For this review, take the finished solid that the model builds, in its own axes (mm). Coordinates: 2 decimals unless noted, no trailing zeros. Loops run counter-clockwise (first coordinate to the right, second up) from the corner with the lowest first, then second, coordinate; pieces in that order, holes last. Notation, with made-up numbers: (43, 43) -> (75, 43) arc R22 ccw to (75, 69) -> close; hole circle Ø3 at (70, 79). An arc over 180 degrees is marked (long way). Use a Markdown table: item, result.
from build123d import *

# Parameters (mm, degrees)
IZIM1_W                     = 80
IZIM1_H                     = 12.7
Y_KSEKLIK_EKSTR_ZYON1_DEPTH = 12.7
IZIM2_R                     = 2.5
IZIM2_R_2                   = 2
KES_EKSTR_ZYON1_DEPTH       = 12.7
KES_EKSTR_ZYON2_DEPTH       = 19.7


with BuildPart() as part:
    # Çizim1 → Yükseklik-Ekstrüzyon1 (new body)
    with BuildSketch(Plane.XY):
        Rectangle(IZIM1_W, IZIM1_H)
    extrude(amount=Y_KSEKLIK_EKSTR_ZYON1_DEPTH)

    # Çizim2 → Kes-Ekstrüzyon1 (cut)
    with BuildSketch(Plane.XY.offset(12.7)):
        with Locations((35, 0)):
            Circle(IZIM2_R)
        with Locations((20, 0)):
            Circle(IZIM2_R)
        with Locations((-35, 0)):
            Circle(IZIM2_R_2)
        with Locations((-20, 0)):
            Circle(IZIM2_R_2)
    extrude(amount=-KES_EKSTR_ZYON1_DEPTH, mode=Mode.SUBTRACT)

    # Çizim3 → Kes-Ekstrüzyon2 (cut)
    with BuildSketch(Plane(origin=(0, 6.35, 0), x_dir=(1, 0, 0), z_dir=(0, 1, 0))):
        with BuildLine():
            ThreePointArc((0, -2.019872981), (-7.5, -6.35), (0, -10.680127019))
            ThreePointArc((0, -10.680127019), (7.5, -6.35), (0, -2.019872981))
        make_face()
    extrude(amount=-KES_EKSTR_ZYON2_DEPTH, mode=Mode.SUBTRACT)


solid = part.part
(1) Take a section at C-C on y = 0. Write out the cut boundary in (x, z), plus the area to 3 significant figures.
Found:
| item | result |
|---|---|
| outline | (-40, 0) -> (-37, 0) -> (-37, 12.7) -> (-40, 12.7) -> close; (-33, 0) -> (-22, 0) -> (-22, 12.7) -> (-33, 12.7) -> close; (-18, 0) -> (17.5, 0) -> (17.5, 12.7) -> (-18, 12.7) -> close; (22.5, 0) -> (32.5, 0) -> (32.5, 12.7) -> (22.5, 12.7) -> close; (37.5, 0) -> (40, 0) -> (40, 12.7) -> (37.5, 12.7) -> close; hole (0, 2.02) arc R5 ccw (long way) to (0, 10.68) arc R5 ccw (long way) to start |
| area | 661 mm^2 |
(2) For line 1 along Y through (x, z) = (20, 6.25); line 2 along Y through (x, z) = (-20, 9); line 3 along Z through (x, y) = (-2.5, 2.75), list the stretches that pass through material, from the lowest coordinate up.
Found:
| item | result |
|---|---|
| line 1 | y = -6.35 to -2.5, 2.5 to 6.35 |
| line 2 | y = -6.35 to -2, 2 to 6.35 |
| line 3 | z = 0 to 1.35, 11.35 to 12.7 |
(3) Take a section at B-B on x = 20. Write out the cut boundary in (y, z).
Found:
| item | result |
|---|---|
| outline | (-6.35, 0) -> (-2.5, 0) -> (-2.5, 12.7) -> (-6.35, 12.7) -> close; (2.5, 0) -> (6.35, 0) -> (6.35, 12.7) -> (2.5, 12.7) -> close |
(4) Take a section at A-A on z = 6.35. Write out the cut boundary in (x, y), plus the area to 3 significant figures.
Found:
| item | result |
|---|---|
| outline | (-40, -6.35) -> (-7.5, -6.35) -> (-7.5, 6.35) -> (-40, 6.35) -> close; (7.5, -6.35) -> (40, -6.35) -> (40, 6.35) -> (7.5, 6.35) -> close; hole circle Ø4 at (-35, 0); hole circle Ø4 at (-20, 0); hole circle Ø5 at (20, 0); hole circle Ø5 at (35, 0) |
| area | 761 mm^2 |
(5) Take a section at D-D on x = -2.5. Write out the cut boundary in (y, z), plus the area to 3 significant figures.
Found:
| item | result |
|---|---|
| outline | (-6.35, 0) -> (6.35, 0) -> (6.35, 1.35) -> (-6.35, 1.35) -> close; (-6.35, 11.35) -> (6.35, 11.35) -> (6.35, 12.7) -> (-6.35, 12.7) -> close |
| area | 34.3 mm^2 |
(6) Mouldability with a two-part tool opening along X and no side actions: class faces 1 (the face through (-1, -6.35, 12)), 2 (the face through (40, 0, 6)), 3 (the face through (-33.153, -0.766, 6.439)) as pulls with the +X half, pulls with the -X half, needs draft (parallel to the pull), parting line crosses it, or undercut.
Found:
| item | result |
|---|---|
| face 1 | needs draft |
| face 2 | pulls with the +X half |
| face 3 | undercut |
